Read the model definition and answer for the solid it produces. Units are mm, in the model's axes. Coordinates: 2 decimals unless noted, no trailing zeros. Loops run counter-clockwise (first coordinate to the right, second up) from the corner with the lowest first, then second, coordinate; pieces in that order, holes last.
Q1. Straight lines are drawn through the part: line 1 (Z direction, x = -46, y = 0.5); line 2 (X direction, y = 8.5, z = -4.5). For each, find the intervals that lie inside material, in ascending order.
Q2. Section A-A (z = -38) is taken. Give the vertices of the cut face in (x, y), then the cut area to 3 significant figures.
Q3. Flat-ended cylindrical pins translate along their axes: P1, Ø5, axis at y = 5.5, z = -95, coming from the -X side; P2, Ø5, axis at y = 3.5, z = -149.5, coming from the +X side; P3, Ø1.5, axis at y = 4.5, z = 3.5, coming from the -X side; P4, Ø10, axis at x = -115, z = -136.5, coming from the -Y side. Find the tip coordinate at first contact, or state that the pin passes through.
Q4. Section B-B (x = -46) is taken. Give the vertices of the cut face in (y, z).
from build123d import *

# Parameters (mm, degrees)
SKETCH2_W           = 180
SKETCH2_H           = 180
BOSS_EXTRUDE1_DEPTH = 10
SKETCH9_W           = 14
SKETCH9_H           = 14
CUT_EXTRUDE2_DEPTH  = 10
SKETCH10_W          = 10
SKETCH10_H          = 10
BOSS_EXTRUDE2_DEPTH = 10
SKETCH11_W          = 10
SKETCH11_H          = 10
CUT_EXTRUDE3_DEPTH  = 10


with BuildPart() as part:
    # Sketch2 → Boss-Extrude1 (new body)
    with BuildSketch(Plane(origin=(0, 0, 0), x_dir=(1, 0, 0), z_dir=(0, 1, 0))):
        with Locations((-90, 90)):
            Rectangle(SKETCH2_W, SKETCH2_H)
    extrude(amount=BOSS_EXTRUDE1_DEPTH)

    # Sketch9 → Cut-Extrude2 (cut)
    with BuildSketch(Plane(origin=(0, 10, 0), x_dir=(1, 0, 0), z_dir=(0, 1, 0))):
        Rectangle(SKETCH9_W, SKETCH9_H)
        with Locations((-180, 0)):
            Rectangle(SKETCH9_W, SKETCH9_H)
        with Locations((-180, 180)):
            Rectangle(SKETCH9_W, SKETCH9_H)
        with Locations((0, 180)):
            Rectangle(SKETCH9_W, SKETCH9_H)
    extrude(amount=-CUT_EXTRUDE2_DEPTH, mode=Mode.SUBTRACT)

    # Sketch10 → Boss-Extrude2 (add)
    with BuildSketch(Plane(origin=(0, 10, 0), x_dir=(1, 0, 0), z_dir=(0, 1, 0))):
        with Locations((-180, 118)):
            Rectangle(SKETCH10_W, SKETCH10_H)
        with Locations((0, 62)):
            Rectangle(SKETCH10_W, SKETCH10_H)
        with Locations((-118, 0)):
            Rectangle(SKETCH10_W, SKETCH10_H)
        with Locations((-62, 180)):
            Rectangle(SKETCH10_W, SKETCH10_H)
    extrude(amount=-BOSS_EXTRUDE2_DEPTH)

    # Sketch11 → Cut-Extrude3 (cut)
    with BuildSketch(Plane(origin=(0, 10, 10), x_dir=(1, 0, 0), z_dir=(0, 1, 0))):
        with Locations((-180, 72)):
            Rectangle(SKETCH11_W, SKETCH11_H)
        with Locations((-62, 10)):
            Rectangle(SKETCH11_W, SKETCH11_H)
        with Locations((-118, 190)):
            Rectangle(SKETCH11_W, SKETCH11_H)
        with Locations((0, 128)):
            Rectangle(SKETCH11_W, SKETCH11_H)
    extrude(amount=-CUT_EXTRUDE3_DEPTH, mode=Mode.SUBTRACT)


solid = part.part
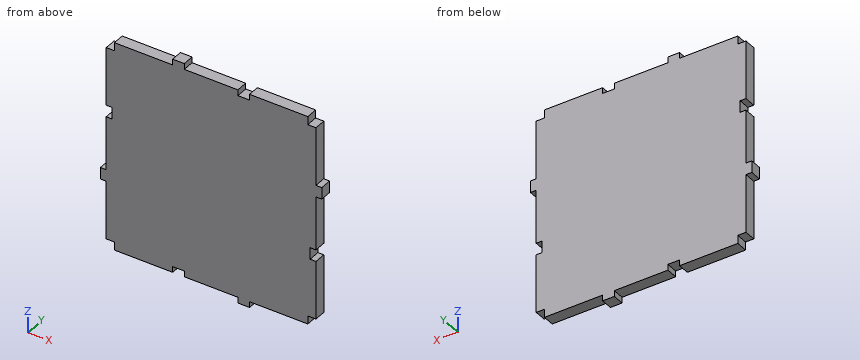
Numbers:
1. line 1: z = -180 to 0
1. line 2: x = -173 to -67, -57 to -7
2. outline: (-180, 0) - (0, 0) - (0, 10) - (-180, 10) - close
2. area: 1,800 mm2
3. P1: stops at x = -180
3. P2: stops at x = 0
3. P3: stops at x = -123
3. P4: stops at y = 0
4. outline: (0, -180) - (10, -180) - (10, 0) - (0, 0) - close
